The model under review builds one solid part; all positions refer to its coordinate system, in mm. A direction names the side the tool comes from. Give positions to 0.01 mm unless a question says otherwise; leave off trailing zeros. Order: outer loops, then holes, each group sorted by start corner. A loop starts at its lowest first (then second) coordinate and runs counter-clockwise, first axis right, second up. Notation, with made-up numbers: (48.5, -40) - (100.5, -40) arc R35 cw to (100.5, -3) - close; hole circle Ø9 at (52.5, 31.25). An arc over 180 degrees is marked (long way). Put each result on its own line as item: value.
Autodesk Inventor part; units mm, degrees
ref_plane "YZ Plane" through (0, 0, 0) normal (1, 0, 0) x (0, 1, 0)
ref_plane "XZ Plane" through (0, 0, 0) normal (0, 1, 0) x (-1, 0, 0)
ref_plane "XY Plane" through (0, 0, 0) normal (0, 0, 1) x (1, 0, 0)
sketch "Эскиз1" plane through (0, 0, 0) normal (0, 1, 0) x (-1, 0, 0)
  line L0 (0, 0) -> (40, 0)
  line L1 (40, 0) -> (40, -40)
  line L2 (40, -40) -> (0, -40)
  line L3 (0, -40) -> (0, 0)
  line L4 (40, 0) -> (40, -2)
  line L5 (0, -40) -> (2, -40)
  line L6 (40, -2) -> (2, -40)
  dimension "d0" = 40
  dimension "d1" = 40
  dimension "d2" = 2
  dimension "d3" = 2
extrude "Выдавливание1" add sketch "Эскиз1" along normal blind 17 contours L0 L1 L6 L2 L3
sketch "Эскиз2" plane through (0, 0, -40) normal (0, 0, -1) x (-1, 0, 0)
  line L0 (0, 17) -> (2, 17)
  line L1 (2, 17) -> (2, 15)
  line L2 (2, 0) -> (2, 17)
  line L3 (2, 15) -> (40, 15)
  line L4 (40, 0) -> (40, 17)
  line L5 (0, 0) -> (2, 0)
  line L6 (2, 0) -> (2, 2)
  line L7 (2, 2) -> (40, 2)
  line L8 (40, 2) -> (40, 15)
  line L9 (2, 15) -> (2, 2)
  dimension "d6" = 2
  dimension "d7" = 2
extrude "Выдавливание2" cut sketch "Эскиз2" against normal blind 38
sketch "Эскиз3" plane through (0, 0, -2) normal (0, 0, -1) x (-1, 0, 0)
  line L0 (0, 0) -> (0, 17)
  line L1 (20, 10.2321) -> (20, 10.5)
  line L2 (20, 10.5) -> (21, 10.5)
  line L3 (21, 6.5) -> (19, 6.5)
  line L4 (19, 10.5) -> (20, 10.5)
  arc A0 (21, 6.5) -> (21, 10.5) centre (21, 8.5) ccw
  arc A1 (19, 10.5) -> (19, 6.5) centre (19, 8.5) ccw
  line L5 (20, 10.5) -> (20, 8.5)
  line L6 (0, 8.5) -> (17, 8.5)
  line L7 (19, 8.5) -> (20, 8.5)
  dimension "d10" = 20
  dimension "d11" = 2
  dimension "d13" = 1
extrude "Выдавливание3" cut sketch "Эскиз3" against normal blind 10
sketch "Эскиз4" plane through (-2, 2, -40) normal (-1, 0, 0) x (0, 0, 1)
  line L0 (0, 0) -> (0, 13)
  line L1 (0, 6.5) -> (20, 6.5)
  line L2 (20, 8.2321) -> (20, 8.5)
  line L3 (20, 8.5) -> (21, 8.5)
  line L4 (21, 4.5) -> (20, 4.5)
  line L5 (20, 4.5) -> (19, 4.5)
  line L6 (19, 8.5) -> (20, 8.5)
  arc A0 (21, 4.5) -> (21, 8.5) centre (21, 6.5) ccw
  arc A1 (19, 8.5) -> (19, 4.5) centre (19, 6.5) ccw
  point P0 (40, -2)
  dimension "d17" = 20
extrude "Выдавливание5" cut sketch "Эскиз4" against normal blind 18.75
properties part number "угол"
(1) Take a section at D-D, the plane y = 4.75. Write out the cut boundary in (x, z).
The answers:
outline: (-40, -2) - (-2, -2) - (-2, -40) - (0, -40) - (0, 0) - (-40, 0) - close
(2) The part is to be moulded in two halves that separate along Y. For faces 6 (the flat face through (-15, 0, -15)), 7 (the flat face through (0, 6, -20)), 8 (the cylindrical face through (-17, 8.5, -1)), say which applies: pulls with the +Y half, pulls with the -Y half, needs draft (parallel to the pull), parting line crosses it, or undercut.
The answers:
face 6: pulls with the -Y half
face 7: needs draft
face 8: undercut
(3) Clearance check with flat-ended pins moving along their axes: pin 1 Ø3 at (x, y) = (-10, 11.5) entering from -Z; pin 2 Ø6.5 at (y, z) = (7.5, -14.5) entering from -X. State where each tip first meets the part, or that it passes through.
The answers:
pin 1: z = -2
pin 2: x = -2
(4) For faces 1 (the flat face through (-20, 10.5, -1)), 2 (the flat face through (-15, 17, -15)), 3 (the flat face through (-21, 11, -2)), 4 (the flat face through (-1, 8, -40)), 5 (the cylindrical face through (-1, 8.5, -23)), list the 3-axis set-ups (+Z, -Z, +X, -X, +Y, -Y) from which the entire face can be reached by the end or side of a thin tool; tool diameter is ignored.
The answers:
face 1: +Z, -Z
face 2: +Z, -Z, +X, -X, +Y
face 3: -Z, -X
face 4: -Z, +X, -X, +Y, -Y
face 5: +X, -X
(5) Take a section at B-B, the plane z = -6.5. Write out the cut boundary in (x, y), then the cut area to 3 significant figures.
The answers:
outline: (-35.5, 0) - (0, 0) - (0, 17) - (-35.5, 17) - (-35.5, 15) - (-2, 15) - (-2, 2) - (-35.5, 2) - close
area: 168 mm^2
(6) Take a section at C-C, the plane x = -12. Write out the cut boundary in (y, z).
The answers:
outline: (0, -30) - (2, -30) - (2, -2) - (15, -2) - (15, -30) - (17, -30) - (17, 0) - (0, 0) - close
(7) Wall thickness on L1, parallel to Y at x = -6.5, z = -10; L2, parallel to Z at x = -26.5, y = 7: over which ranges is each line inside the solid? List them lowest first.
The answers:
L1: 0 to 2, 15 to 17
L2: -2 to 0
(8) Take a section at A-A, the plane y = 9.25. Write out the cut boundary in (x, z), then the cut area to 3 significant figures.
The answers:
outline: (-40, -2) - (-22.85, -2) - (-22.85, 0) - (-40, 0) - close; (-17.15, -2) - (-2, -2) - (-2, -17.15) - (0, -17.15) - (0, 0) - (-17.15, 0) - close; (-2, -40) - (0, -40) - (0, -22.85) - (-2, -22.85) - close
area: 133 mm^2
